Can you work these out from the model? Positions are in its coordinate system, mm. A direction names the side the tool comes from. Round coordinates to 2 decimals unless told otherwise and drop trailing zeros. Order: outer loops, then holes, each group sorted by start corner. A loop starts at its lowest first (then second) coordinate and runs counter-clockwise, first axis right, second up.
from build123d import *

# Parameters (mm, degrees)
SKETCH1_R               = 1.7
SKETCH1_R_2             = 1.6
BOSS_EXTRUDE1_DEPTH     = 22
CUT_EXTRUDE1_DEPTH      = 6
CUT_EXTRUDE2_START      = -2
CUT_EXTRUDE2_DEPTH      = 5
CHAMFER1_SIZE           = 3
CHAMFER1_SIZE2          = 8.242432258
SKETCH4_R               = 2.2
SKETCH4_R_2             = 1.6
BOSS_EXTRUDE2_DEPTH     = 0.15
SKETCH5_R               = 7.371028059
CUT_EXTRUDE3_DEPTH      = 0.25
FILLET1_R               = 1
CUT_EXTRUDE4_DEPTH      = 12.25
CUT_EXTRUDE4_DEPTH_BACK = 4.75
SKETCH8_W               = 8
SKETCH8_H               = 3
BOSS_EXTRUDE4_DEPTH     = 1
SKETCH10_R              = 1.25
CUT_EXTRUDE7_DEPTH      = 4
SKETCH11_W              = 5
SKETCH11_H              = 3
BOSS_EXTRUDE5_DEPTH     = 1


with BuildPart() as part:
    # Sketch1 → Boss-Extrude1 (new body)
    with BuildSketch(Plane(origin=(0, 0, 0), x_dir=(0, 0, -1), z_dir=(1, 0, 0))):
        with BuildLine():
            Line((-3.247595264, 1.875), (1.082531755, 9.375))
            ThreePointArc((1.082531755, 9.375), (2.455127019, 10.747595264), (4.330127019, 11.25))
            Line((4.330127019, 11.25), (15, 11.25))
            Line((15, 11.25), (15, 3.75))
            Line((15, 3.75), (6.495190528, 3.75))
            Line((6.495190528, 3.75), (3.247595264, -1.875))
            ThreePointArc((3.247595264, -1.875), (-1.875, -3.247595264), (-3.247595264, 1.875))
        make_face()
        Circle(SKETCH1_R, mode=Mode.SUBTRACT)
        with Locations((4.330127019, 7.5)):
            Circle(SKETCH1_R_2, mode=Mode.SUBTRACT)
    extrude(amount=BOSS_EXTRUDE1_DEPTH)

    # Sketch2 → Cut-Extrude1 (cut)
    with BuildSketch(Plane.ZY):
        Polygon((-15, 11.25), (5.328677025, 11.25), (5.328677025, -6.255762667), (0, -6.255762667), (0, 0), (-1.299038106, 2.25), (-5.629165125, 2.25), (-15, 2.25), align=None)
    extrude(amount=-CUT_EXTRUDE1_DEPTH, mode=Mode.SUBTRACT)

    # Sketch3 → Cut-Extrude2 (cut)
    with BuildSketch(Plane(origin=(0, 0, -15), x_dir=(-1, 0, 0), z_dir=(0, 0, -1)).offset(CUT_EXTRUDE2_START)):
        with BuildLine():
            Line((-19.5, 3.75), (-19.5, 5.15))
            ThreePointArc((-19.5, 5.15), (-19.03137085, 6.28137085), (-17.9, 6.75))
            Line((-17.9, 6.75), (-10.1, 6.75))
            Line((-10.1, 6.75), (-6, 6.75))
            Line((-6, 6.75), (-6, 3.75))
            Line((-6, 3.75), (-8.5, 3.75))
            Line((-8.5, 3.75), (-19.5, 3.75))
        make_face()
    extrude(amount=-CUT_EXTRUDE2_DEPTH, mode=Mode.SUBTRACT)

    # Chamfer1
    chamfer1_edges = [part.edges().sort_by_distance(p)[0] for p in [
        (14, 11.25, -15),
    ]]
    chamfer1_side = [part.faces().sort_by_distance(p)[0] for p in [
        (14, 7.5, -15),
    ]]
    chamfer(chamfer1_edges, length=CHAMFER1_SIZE, length2=CHAMFER1_SIZE2, reference=chamfer1_side[0])

    # Sketch4 → Boss-Extrude2 (add)
    with BuildSketch(Plane.ZY.offset(-6)):
        with Locations((-4.330127019, 7.5)):
            Circle(SKETCH4_R)
        with Locations((-4.330127019, 7.5)):
            Circle(SKETCH4_R_2, mode=Mode.SUBTRACT)
    extrude(amount=BOSS_EXTRUDE2_DEPTH)

    # Sketch5 → Cut-Extrude3 (cut)
    with BuildSketch(Plane.ZY):
        Circle(SKETCH5_R)
    extrude(amount=-CUT_EXTRUDE3_DEPTH, mode=Mode.SUBTRACT)

    # Fillet1
    fillet1_edges = [part.edges().sort_by_distance(p)[0] for p in [
        (3.125, 2.25, -5.629165125),
        (14, 3.75, -15),
        (14, 3.75, -6.495190528),
        (14, 8.25, -15),
    ]]
    fillet(fillet1_edges, radius=FILLET1_R)

    # Sketch7 → Cut-Extrude4 (cut, two sides)
    with BuildSketch(Plane(origin=(0, 0, 0), x_dir=(1, 0, 0), z_dir=(0, 1, 0))) as cut_extrude4_sk:
        Polygon((22, 4), (14, 15), (22, 15), align=None)
    extrude(amount=CUT_EXTRUDE4_DEPTH, mode=Mode.SUBTRACT)
    extrude(cut_extrude4_sk.sketch, amount=-CUT_EXTRUDE4_DEPTH_BACK, mode=Mode.SUBTRACT)

    # Sketch8 → Boss-Extrude4 (add)
    with BuildSketch(Plane(origin=(16.291891892, 0, -11.848648649), x_dir=(-0.588171698, 0, -0.808736084), z_dir=(0.808736084, 0, -0.588171698))):
        with Locations((-1.339859822, 5.25)):
            Rectangle(SKETCH8_W, SKETCH8_H)
    extrude(amount=-BOSS_EXTRUDE4_DEPTH)

    # Sketch10 → Cut-Extrude7 (cut)
    with BuildSketch(Plane(origin=(0, 1.875, 3.247595264), x_dir=(1, 0, 0), z_dir=(0, 0.5, 0.866025404))):
        with Locations((14, 8.660254038)):
            Circle(SKETCH10_R)
    extrude(amount=-CUT_EXTRUDE7_DEPTH, mode=Mode.SUBTRACT)

    # Sketch11 → Boss-Extrude5 (add)
    with BuildSketch(Plane.ZY.offset(-6)):
        with Locations((-10.5, 5.25)):
            Rectangle(SKETCH11_W, SKETCH11_H)
    extrude(amount=-BOSS_EXTRUDE5_DEPTH)


solid = part.part
(1) I want a section at B-B, the plane x = 16.5. Give the number of separate pieces and of enclosed holes in the cut face, plus the area to 3 significant figures.
(2) I want a section at A-A, the plane y = 0. List the corners of the cut face in (x, z) for me.
(3) If we mould it in two halves opening along Z, with no side actions, what happens to faces 5 (the face through (14, 11.25, -6)), 6 (the face through (11, 6.75, -11)), 7 (the face through (10.425, 4.051, -14.715))? For each: pulls with the +Z half, pulls with the -Z half, needs draft (parallel to the pull), parting line crosses it, or undercut.
(4) I want a section at C-C, the plane z = -11.5. List the corners of the cut face in (x, y) for me, plus the area to 3 significant figures.
(5) On a 3-axis mill with a long thin cutter (end or side, diameter ignored), from which of +Z, -Z, +X, -X, +Y, -Y can I reach the whole of each face in a straight line? I mean faces 1 (the face through (3, -3, 0)), 2 (the face through (5.85, 6, -3)), 3 (the face through (3.085, 1.763, -4.756)), 4 (the face through (16.062, 5.271, -10.465)). Say none if no direction works.
(6) Please list where these lines run through material, in increasing order: probe 1 along Z at (x, y) = (9.75, 7.5); probe 2 along Z at (x, y) = (5, 0); probe 3 along Y at (x, z) = (8.5, 1).
(7) I'm going to push flat-ended pins straight in: pin 1 Ø1.5 at (x, y) = (10.5, 5.5) entering from +Z; pin 2 Ø2 at (y, z) = (6.5, -5) entering from -X; pin 3 Ø3.5 at (x, z) = (14, -11) entering from -Y. Where does each tip first touch, or does it pass through?
Ans:
1. separate pieces: 1
1. enclosed holes: 2
1. area: 114 mm2
2. outline: (0.25, -4.33) - (21.76, -4.33) - (22, -4) - (22, -1.7) - (0.25, -1.7) - close; (6, 1.7) - (22, 1.7) - (22, 3.75) - (6, 3.75) - close
3. face 5: needs draft
3. face 6: undercut
3. face 7: pulls with the -Z half
4. outline: (6, 3.75) - (7, 3.75) - (7, 6.75) - (15.31, 6.75) - (15.31, 3.75) - (16.55, 3.75) - (16.55, 9.52) - (6, 9.52) - close
4. area: 36.0 mm2
5. face 1: +Z, -X, +Y, -Y
5. face 2: +Z, -Z, -X, +Y
5. face 3: -Z, -X
5. face 4: -Y
6. probe 1: z = -15 to -5.93, -2.73 to 0
6. probe 2: z = -4.33 to -1.7
6. probe 3: y = -3.61 to -1.37, 1.37 to 5.77
7. pin 1: stops at z = 1.59
7. pin 2: stops at x = 5.85
7. pin 3: stops at y = 3.75
